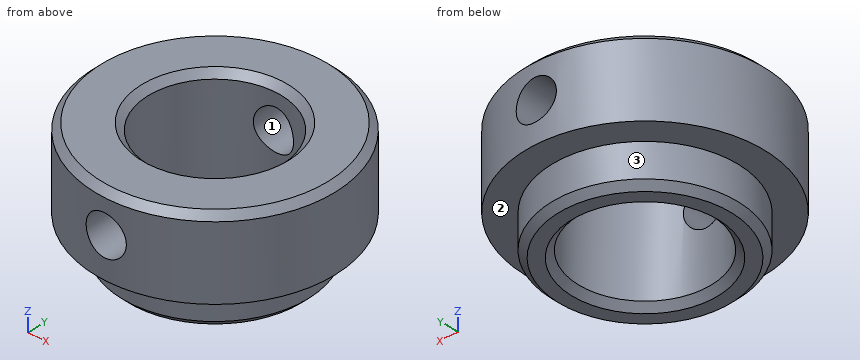
from build123d import *

# Parameters (mm, degrees)
F0_R     = 7
F0_R_2   = 5
F1_DEPTH = 3
F2_R     = 9
F2_R_2   = 5
F3_DEPTH = 6
F4_R     = 1.5
F5_DEPTH = 12.5
F6_SIZE  = 0.5


with BuildPart() as f1:
    # F0 (on Top) → F1 (new body)
    with BuildSketch(Plane.XY):
        Circle(F0_R)
        Circle(F0_R_2, mode=Mode.SUBTRACT)
    extrude(amount=F1_DEPTH)

    # F2 (on face) → F3 (join)
    with BuildSketch(Plane.XY.offset(3)):
        Circle(F2_R)
        Circle(F2_R_2, mode=Mode.SUBTRACT)
    extrude(amount=F3_DEPTH)

    # F4 (on Front) → F5 (cut, symmetric)
    with BuildSketch(Plane.XZ):
        with Locations((0, 6)):
            Circle(F4_R)
    extrude(amount=F5_DEPTH, both=True, mode=Mode.SUBTRACT)

    # F6
    f6_edges = [f1.edges().sort_by_distance(p)[0] for p in [
        (-9, 0, 9),
        (-7, 0, 0),
        (-5, 0, 9),
        (-5, 0, 0),
    ]]
    chamfer(f6_edges, length=F6_SIZE)


solid = f1.part
Can you work these out from the model? Positions are in its coordinate system, mm. Face numbers are marked on the shaded views. Give positions to 0.01 mm unless a question says otherwise; leave off trailing zeros. Loops run counter-clockwise (first coordinate to the right, second up) from the corner with the lowest first, then second, coordinate; pieces in that order, holes last. Notation, with made-up numbers: (39.5, -37) - (59.5, -37) arc R24 ccw to (59.5, -7) - close; hole circle Ø3 at (57.25, 83). An arc over 180 degrees is marked (long way). One line per item, written item: value.
(1) If we mould it in two halves opening along X, with no side actions, what happens to the marked faces 1, 2 and 3? For each: released by +X, released by -X, zero draft, split by the parting line, or undercut.
Verdict:
face 1: undercut
face 2: zero draft
face 3: split by the parting line
(2) If we section it at D-D, the plane z = 4: List the corners of the cut face in (x, y) for me.
Verdict:
outline: circle Ø18 at (0, 0); hole circle Ø10 at (0, 0)
(3) I'm going to push a flat-ended pin straight in: pin 1 (2 mm diameter, centred on y = -5.5, z = 3, fed in from +X). Where does the tip first touch, or does it pass through?
Verdict:
pin 1: x = 7.79
(4) If we section it at A-A, the plane x = 0: List the corners of the cut face in (y, z) for me, plus the area to 3 significant figures.
Verdict:
outline: (-9, 3) - (-7, 3) - (-7, 0.5) - (-6.5, 0) - (-5.5, 0) - (-5, 0.5) - (-5, 4.5) - (-9, 4.5) - close; (-9, 7.5) - (-5, 7.5) - (-5, 8.5) - (-5.5, 9) - (-8.5, 9) - (-9, 8.5) - close; (5, 0.5) - (5.5, 0) - (6.5, 0) - (7, 0.5) - (7, 3) - (9, 3) - (9, 4.5) - (5, 4.5) - close; (5, 7.5) - (9, 7.5) - (9, 8.5) - (8.5, 9) - (5.5, 9) - (5, 8.5) - close
area: 35.0 mm^2
(5) If we section it at C-C, the plane z = 6: List the corners of the cut face in (x, y) for me.
Verdict:
outline: (-1.5, -8.87) - (-1.5, -4.77) arc R5 cw to (-1.5, 4.77) - (-1.5, 8.87) arc R9 ccw to start; (1.5, -8.87) arc R9 ccw to (1.5, 8.87) - (1.5, 4.77) arc R5 cw to (1.5, -4.77) - close
(6) If we section it at B-B, the plane y = 0: List the corners of the cut face in (x, z) for me, plus the area to 3 significant figures.
Verdict:
outline: (-9, 3) - (-7, 3) - (-7, 0.5) - (-6.5, 0) - (-5.5, 0) - (-5, 0.5) - (-5, 8.5) - (-5.5, 9) - (-8.5, 9) - (-9, 8.5) - close; (5, 0.5) - (5.5, 0) - (6.5, 0) - (7, 0.5) - (7, 3) - (9, 3) - (9, 8.5) - (8.5, 9) - (5.5, 9) - (5, 8.5) - close
area: 59.0 mm^2
(7) I need wall thicknesses on line 1 along Z through (x, y) = (0, -5.95); line 2 along Z through (x, y) = (0, 7.6); line 3 along X through (y, z) = (5.75, 5). Which ranges of each line are inside material? Lowest first, please.
Verdict:
line 1: 0 to 4.5, 7.5 to 9
line 2: 3 to 4.5, 7.5 to 9
line 3: -6.92 to -1.12, 1.12 to 6.92
